Autodesk Fusion 360 part; units mm, degrees
sketch "Sketch1" plane through (0, 0, 0) normal (0, 0, 1) x (1, 0, 0)
  line L0 (0, 0) -> (75, 0)
  line L1 (75, 0) -> (75, 12.7)
  line L2 (75, 12.7) -> (0, 12.7)
  line L3 (0, 12.7) -> (0, 0)
  dimension "d1" = 75
  dimension "d2" = 12.7
extrude "Extrude1" add sketch "Sketch1" along normal blind 12.7
sketch "Sketch2" plane through (0, 0, 12.7) normal (0, 0, 1) x (-1, 0, 0)
  line L0 (0, -12.7) -> (0, 0)
  line L1 (0, 0) -> (-75, 0)
  line L2 (-75, 0) -> (-75, -12.7)
  line L3 (-75, -12.7) -> (0, -12.7)
  circle A0 centre (-5.5, -6.35) radius 2
  circle A1 centre (-15.5, -6.35) radius 2
  circle A2 centre (-69.5, -6.35) radius 2
  circle A3 centre (-59.5, -6.35) radius 2
  line L4 (-5.5, -6.35) -> (0, -6.35)
  line L5 (-69.5, -6.35) -> (-75, -6.35)
  dimension "d5" = 4
  dimension "d6" = 4
  dimension "d7" = 10
  dimension "d8" = 4
  dimension "d9" = 4
  dimension "d10" = 10
  dimension "d11" = 44
  dimension "d12" = 64
extrude "Extrude2" cut sketch "Sketch2" against normal blind 17.78 contours A0 | A2 | A1 | A3
thread "Thread1" thread offset 0 thread length 10.0076
Here's how the part is built. I have some questions about the finished solid (model axes, mm). Coordinates: 2 decimals unless noted, no trailing zeros. Order: outer loops, then holes, each group sorted by start corner. A loop starts at its lowest first (then second) coordinate and runs counter-clockwise, first axis right, second up. Notation, with made-up numbers: (41.25, 63.5) - (79.25, 63.5) arc R26 ccw to (79.25, 88.5) - close; hole circle Ø6 at (32.5, 63). An arc over 180 degrees is marked (long way). Use CSV: the item, a comma, the result in double quotes. Start each with the question number.
1. Suppose I cut it at B-B on x = 59.5. List the corners of the cut face in (y, z) for me, then the cut area to 3 significant figures.
2. Suppose I cut it at C-C on z = 4.5. List the corners of the cut face in (x, y) for me.
3. I'm going to push a flat-ended pin straight in: pin 1 (3.5 mm diameter, centred on x = 15.5, y = 6.35, fed in from -Z). Where does the tip first touch, or does it pass through?
4. Please list where these lines run through material, in increasing order: line 1 (X direction, y = 6.35, z = 9.75); line 2 (X direction, y = 7.5, z = 11.75); line 3 (Y direction, x = 69.5, z = 3.5). Write a range as from..to.
5. If we mould it in two halves opening along Y, with no side actions, what happens to faces 1 (the face through (15.76, 4.367, 6.439)), 2 (the face through (0, 6, 6)), 3 (the face through (38, 12.7, 6))? For each: +Y half, -Y half, draft (parallel to the pull), parting line (faces both ways), or undercut.
6. Suppose I cut it at A-A on y = 6.35. List the corners of the cut face in (x, z) for me.
7. Suppose I cut it at D-D on x = 15. List the corners of the cut face in (y, z) for me.
Output:
1,outline,"(0, 0) - (4.35, 0) - (4.35, 12.7) - (0, 12.7) - close; (8.35, 0) - (12.7, 0) - (12.7, 12.7) - (8.35, 12.7) - close"
1,area,"110 mm2"
2,outline,"(0, 0) - (75, 0) - (75, 12.7) - (0, 12.7) - close; hole circle Ø4 at (5.5, 6.35); hole circle Ø4 at (15.5, 6.35); hole circle Ø4 at (59.5, 6.35); hole circle Ø4 at (69.5, 6.35)"
3,pin 1,"passes through"
4,line 1,"x = 0..3.5, 7.5..13.5, 17.5..57.5, 61.5..67.5, 71.5..75"
4,line 2,"x = 0..3.86, 7.14..13.86, 17.14..57.86, 61.14..67.86, 71.14..75"
4,line 3,"y = 0..4.35, 8.35..12.7"
5,face 1,"undercut"
5,face 2,"draft"
5,face 3,"+Y half"
6,outline,"(0, 0) - (3.5, 0) - (3.5, 12.7) - (0, 12.7) - close; (7.5, 0) - (13.5, 0) - (13.5, 12.7) - (7.5, 12.7) - close; (17.5, 0) - (57.5, 0) - (57.5, 12.7) - (17.5, 12.7) - close; (61.5, 0) - (67.5, 0) - (67.5, 12.7) - (61.5, 12.7) - close; (71.5, 0) - (75, 0) - (75, 12.7) - (71.5, 12.7) - close"
7,outline,"(0, 0) - (4.41, 0) - (4.41, 12.7) - (0, 12.7) - close; (8.29, 0) - (12.7, 0) - (12.7, 12.7) - (8.29, 12.7) - close"
